Design review of the part built by this model. Coordinates are the model's own, in mm. A direction names the side the tool comes from. Coordinates: 2 decimals unless noted, no trailing zeros. Loops run counter-clockwise (first coordinate to the right, second up) from the corner with the lowest first, then second, coordinate; pieces in that order, holes last. Notation, with made-up numbers: (19, 68) - (60, 68) arc R18 cw to (60, 81) - close; hole circle Ø10 at (73, 5). An arc over 180 degrees is marked (long way). Use one line per item in the form item = value. Start each with the question number.
(1) Add section A-A (x = 0). State the section outline as (y, z) points.
(2) Tool access review of faces 5 (the face through (0, 2, 4)), 6 (the face through (-0.54, 0.99, 2.44)): name each direction out of +Z, -Z, +X, -X, +Y, -Y from which nothing blocks a thin tool from reaching the whole face with its end or side.
(3) The part is to be moulded in two halves that separate along Z. For faces 1 (the face through (-12, 2, 0)), 2 (the face through (-1.5, 2.99, -0.07)), 3 (the face through (0, 2, 2)), 4 (the face through (11.43, 1.97, 3.4)), say which applies: pulls with the +Z half, pulls with the -Z half, needs draft (parallel to the pull), parting line crosses it, or undercut.
(4) Add section B-B (y = 3.1). State the section outline as (x, z) points.
(5) For L1, parallel to X at y = 1.1, z = 0; L2, parallel to Z at x = 0, y = 2.8; L3, parallel to Z at x = 0, y = 0.75, list the stretches that pass through material, from the lowest coordinate up.
(6) Add section C-C (z = 0). State the section outline as (x, y) points, plus the area to 3 significant figures.
(7) Clearance check with a flat-ended pin moving along its axis: pin 1 Ø2.5 at (x, z) = (7, 0) entering from -Y. State where the tip first meets the part, or that it passes through.
(8) Add section D-D (x = -7). State the section outline as (y, z) points, plus the area to 3 significant figures.
```python
from build123d import *

# Parameters (mm, degrees)
BOSS_EXTRUDE1_DEPTH = 4
CUT_EXTRUDE1_REACH  = 6
SKETCH1_3_R         = 1.5
SKETCH1_4_R         = 2.5
CUT_EXTRUDE2_DEPTH  = 2


with BuildPart() as part:
    # Sketch1 → Boss-Extrude1 (new body)
    with BuildSketch(Plane(origin=(0, 0, 0), x_dir=(1, 0, 0), z_dir=(0, 1, 0))):
        with BuildLine():
            Line((0, 4), (10, 4))
            ThreePointArc((10, 4), (11.414213562, 3.414213562), (12, 2))
            Line((12, 2), (12, -2))
            ThreePointArc((12, -2), (11.414213562, -3.414213562), (10, -4))
            Line((10, -4), (0, -4))
            Line((0, -4), (-10, -4))
            ThreePointArc((-10, -4), (-11.414213562, -3.414213562), (-12, -2))
            Line((-12, -2), (-12, 2))
            ThreePointArc((-12, 2), (-11.414213562, 3.414213562), (-10, 4))
            Line((-10, 4), (0, 4))
        make_face()
    extrude(amount=BOSS_EXTRUDE1_DEPTH)

    # Sketch1_3 → Cut-Extrude1 (cut, up to next)
    with BuildSketch(Plane(origin=(0, 0, 0), x_dir=(1, 0, 0), z_dir=(0, 1, 0)), mode=Mode.PRIVATE) as cut_extrude1_sk1:
        Circle(SKETCH1_3_R)
    cut_extrude1_tool1 = extrude(cut_extrude1_sk1.sketch, amount=CUT_EXTRUDE1_REACH, mode=Mode.PRIVATE) & part.part
    add(cut_extrude1_tool1.solids().sort_by_distance((0, 0, 0))[0], mode=Mode.SUBTRACT)
    # Sketch1_3 → Cut-Extrude1 (cut, up to next)
    with BuildSketch(Plane(origin=(0, 0, 0), x_dir=(1, 0, 0), z_dir=(0, 1, 0)), mode=Mode.PRIVATE) as cut_extrude1_sk2:
        with Locations((-7, 0)):
            Circle(SKETCH1_3_R)
    cut_extrude1_tool2 = extrude(cut_extrude1_sk2.sketch, amount=CUT_EXTRUDE1_REACH, mode=Mode.PRIVATE) & part.part
    add(cut_extrude1_tool2.solids().sort_by_distance((-7, 0, 0))[0], mode=Mode.SUBTRACT)
    # Sketch1_3 → Cut-Extrude1 (cut, up to next)
    with BuildSketch(Plane(origin=(0, 0, 0), x_dir=(1, 0, 0), z_dir=(0, 1, 0)), mode=Mode.PRIVATE) as cut_extrude1_sk3:
        with Locations((7, 0)):
            Circle(SKETCH1_3_R)
    cut_extrude1_tool3 = extrude(cut_extrude1_sk3.sketch, amount=CUT_EXTRUDE1_REACH, mode=Mode.PRIVATE) & part.part
    add(cut_extrude1_tool3.solids().sort_by_distance((7, 0, 0))[0], mode=Mode.SUBTRACT)

    # Sketch1_4 → Cut-Extrude2 (cut)
    with BuildSketch(Plane(origin=(0, 0, 0), x_dir=(1, 0, 0), z_dir=(0, 1, 0))):
        Circle(SKETCH1_4_R)
    extrude(amount=CUT_EXTRUDE2_DEPTH, mode=Mode.SUBTRACT)


solid = part.part
```
Computed values:
q1.outline = (0, -4) - (4, -4) - (4, -1.5) - (2, -1.5) - (2, -2.5) - (0, -2.5) - close; (0, 2.5) - (2, 2.5) - (2, 1.5) - (4, 1.5) - (4, 4) - (0, 4) - close
q2.face_5 = +Z, +X, -X, +Y, -Y
q2.face_6 = -Y
q3.face_1 = needs draft
q3.face_2 = undercut
q3.face_3 = undercut
q3.face_4 = pulls with the +Z half
q4.outline = (-12, -2) arc R2 ccw to (-10, -4) - (10, -4) arc R2 ccw to (12, -2) - (12, 2) arc R2 ccw to (10, 4) - (-10, 4) arc R2 ccw to (-12, 2) - close; hole circle Ø3 at (-7, 0); hole circle Ø3 at (0, 0); hole circle Ø3 at (7, 0)
q5.L1 = -12 to -8.5, -5.5 to -2.5, 2.5 to 5.5, 8.5 to 12
q5.L2 = -4 to -1.5, 1.5 to 4
q5.L3 = -4 to -2.5, 2.5 to 4
q6.outline = (-12, 0) - (-8.5, 0) - (-8.5, 4) - (-12, 4) - close; (-5.5, 0) - (-2.5, 0) - (-2.5, 2) - (-1.5, 2) - (-1.5, 4) - (-5.5, 4) - close; (1.5, 2) - (2.5, 2) - (2.5, 0) - (5.5, 0) - (5.5, 4) - (1.5, 4) - close; (8.5, 0) - (12, 0) - (12, 4) - (8.5, 4) - close
q6.area = 56.0 mm^2
q7.pin_1 = through
q8.outline = (0, -4) - (4, -4) - (4, -1.5) - (0, -1.5) - close; (0, 1.5) - (4, 1.5) - (4, 4) - (0, 4) - close
q8.area = 20.0 mm^2
